Could you check a few things on this model? Use its own coordinates, in mm. Give positions to 0.01 mm unless a question says otherwise; leave off trailing zeros. Order: outer loops, then holes, each group sorted by start corner. A loop starts at its lowest first (then second) coordinate and runs counter-clockwise, first axis right, second up. Notation, with made-up numbers: (19, 16) -> (53, 16) arc R24 ccw to (53, 31) -> close; hole circle Ø9 at (-12.75, 62). An arc over 180 degrees is marked (long way). One line per item, written item: value.
Autodesk Inventor part; units mm, degrees
ref_plane "YZ Plane" through (0, 0, 0) normal (1, 0, 0) x (0, 1, 0)
ref_plane "XZ Plane" through (0, 0, 0) normal (0, 1, 0) x (-1, 0, 0)
ref_plane "XY Plane" through (0, 0, 0) normal (0, 0, 1) x (1, 0, 0)
sketch "Sketch1" plane through (0, 0, 0) normal (1, 0, 0) x (0, 1, 0)
  line L0 (0, 0) -> (0, -609.6)
  line L1 (0, -609.6) -> (426.8465, -609.6)
  line L2 (426.8465, -609.6) -> (0, 0)
  line L3 (25.4, -80.5585) -> (378.0536, -584.2)
  line L4 (378.0536, -584.2) -> (25.4, -584.2)
  line L5 (25.4, -584.2) -> (25.4, -80.5585)
  dimension "d0" = 609.6
  dimension "d1" = 35
  dimension "d2" = 25.4
  dimension "d3" = 25.4
  dimension "d4" = 25.4
extrude "Extrusion1" add sketch "Sketch1" along normal mid plane 25.4
sketch "Sketch4" plane through (12.7, 0, 0) normal (1, 0, 0) x (0, 0, -1)
  line L0 (609.6, 0) -> (609.6, 426.8465)
  line L1 (0, 0) -> (609.6, 426.8465)
  line L2 (584.2, 25.4) -> (80.5585, 25.4)
  line L3 (80.5585, 25.4) -> (609.6, 395.8388)
  line L4 (80.5585, 25.4) -> (44.2835, 0)
  line L5 (0, 0) -> (609.6, 0)
  line L6 (44.2835, 0) -> (0, 0)
  line L7 (609.6, 426.8465) -> (609.6, 395.8388)
extrude "Extrusion3" add sketch "Sketch4" along normal blind 25.4 contours L3 L4 L5 L1 L0
sketch "Sketch2" plane through (-12.7, 0, 0) normal (-1, 0, 0) x (0, 0, 1)
  line L0 (-609.6, 0) -> (-609.6, 426.8465)
  line L1 (-609.6, 426.8465) -> (0, 0)
  line L2 (-609.6, 426.8465) -> (0, 0)
  line L3 (-80.5585, 25.4) -> (-584.2, 378.0536)
  line L4 (-584.2, 378.0536) -> (-39.5154, 0)
  line L5 (0, 0) -> (-609.6, 0)
  line L6 (-584.2, 378.0536) -> (-609.6, 395.8388)
  line L7 (-609.6, 511.5151) -> (-609.6, 395.8388)
  line L8 (-39.5154, 0) -> (0, 0)
  point P0 (-69.7859, 25.4)
properties part number "ballRampRightSide-35degree-V04"
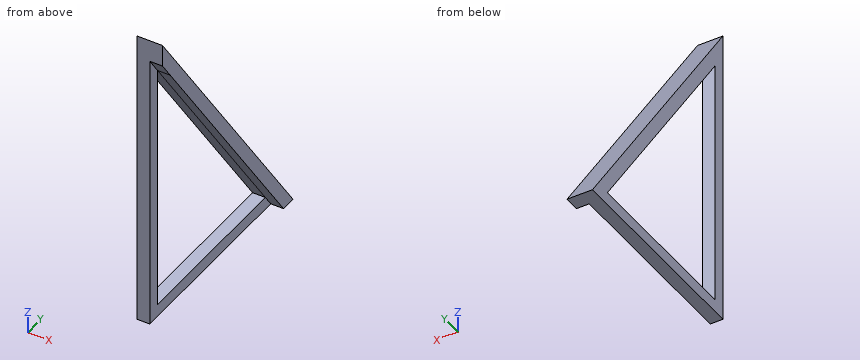
1) Suppose I cut it at B-B, the plane x = -6.5. Write out the boundary of the cut face in (y, z).
Answer below:
outline: (0, -609.6) -> (426.85, -609.6) -> (0, 0) -> close; hole (25.4, -584.2) -> (378.05, -584.2) -> (25.4, -80.56) -> close
2) For P1, Ø1.5, axis at x = 3, z = -418.5, coming from the +Y side; P2, Ø12, axis at x = 3, z = -247, coming from the +Y side; P3, Ø7.5, axis at x = -5.5, z = -319, coming from the +Y side, each with a flat end and sliding along its axis, tell me the tip position at first contact or that it passes through.
Answer below:
P1: stops at y = 293.56
P2: stops at y = 177.15
P3: stops at y = 225.99
3) If I drill on line 1 along Z through (x, y) = (5.5, 291.5); line 2 along Y through (x, z) = (9, -536); line 3 along Z through (x, y) = (-4.5, 210.5), over which ranges is the centre line in solid material (lowest first)?
Answer below:
line 1: z = -609.6 to -584.2, -460.59 to -416.31
line 2: y = 0 to 25.4, 344.3 to 375.31
line 3: z = -609.6 to -584.2, -344.91 to -300.63
